Geometry: final body of the model. Coordinates: model frame, mm. Face numbers are marked on the shaded views. A direction names the side the tool comes from. Coordinates: 2 decimals unless noted, no trailing zeros. Loops run counter-clockwise (first coordinate to the right, second up) from the corner with the lowest first, then second, coordinate; pieces in that order, holes last. Notation, with made-up numbers: (34, -23.75) - (74, -23.75) arc R23 ccw to (74, 1.25) - close; hole circle Ø8 at (43.25, 27.25). An arc over 180 degrees is marked (long way). Answer in a Markdown table with one row per item.
from build123d import *

# Parameters (mm, degrees)
F0_W     = 50.8
F0_H     = 50.8
F0_R     = 2.8336716143
F1_DEPTH = 127
F4_R     = 2.3649720561
F5_DEPTH = 50.8
F5_TAPER = 2
F0_W_2   = 43.18
F0_H_2   = 38.1
F6_DEPTH = 41.91


with BuildPart() as f1:
    # F0 (on Top) → F1 (new body)
    with BuildSketch(Plane.XY):
        Rectangle(F0_W, F0_H)
        Circle(F0_R, mode=Mode.SUBTRACT)
    extrude(amount=F1_DEPTH)

    # F2 (on Front) → F3 (revolve)
    with BuildSketch(Plane.XZ):
        with BuildLine():
            Line((0, 108.9572302283), (0, 144.6343966542))
            ThreePointArc((0, 144.6343966542), (-17.8385832129, 126.7958134413), (0, 108.9572302283))
        make_face()
    revolve(axis=Axis((0, 0, 74.6575031662), (0, 0, -1)))

    # F4 (on face) → F5 (join)
    with BuildSketch(Plane.XY.offset(127)):
        Circle(F4_R)
    extrude(amount=F5_DEPTH, taper=F5_TAPER)

    # F0 (on Top) → F6 (join)
    with BuildSketch(Plane.XY):
        Rectangle(F0_W, F0_H)
        Circle(F0_R, mode=Mode.SUBTRACT)
        with Locations((46.99, 0)):
            Rectangle(F0_W_2, F0_H)
        with Locations((46.99, 44.45)):
            Rectangle(F0_W_2, F0_H_2)
    extrude(amount=F6_DEPTH)

    # F7 (on Front) → F8 (revolve)
    with BuildSketch(Plane.XZ):
        with BuildLine():
            Line((44.333525002, 29.0094343104), (44.333525002, 54.918085309))
            ThreePointArc((44.333525002, 54.918085309), (31.3791995027, 41.9637598097), (44.333525002, 29.0094343104))
        make_face()
    revolve(axis=Axis((44.333525002, 0, 30.4748073686), (0, 0, -1)))


solid = f1.part
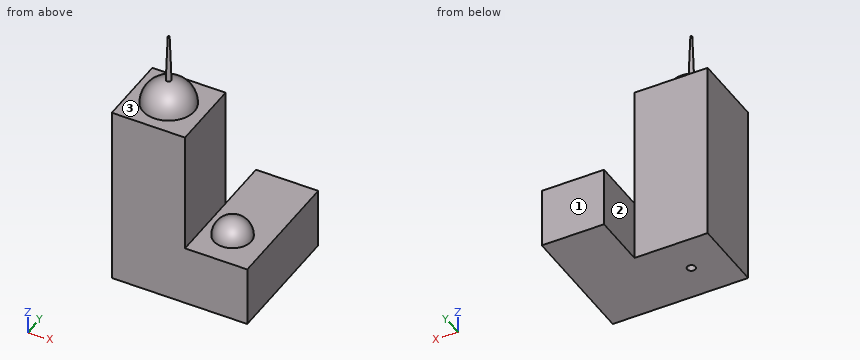
(1) Cut plane A-A on z = 72. Output: boundary loops of the cut face in (x, y), then the cut area to 3 significant figures.
Verdict:
| item | result |
|---|---|
| outline | (-25.4, -25.4) - (25.4, -25.4) - (25.4, 25.4) - (-25.4, 25.4) - close; hole circle Ø5.67 at (0, 0) |
| area | 2,560 mm² |
(2) First-contact query: pin 1 Ø8 at (y, z) = (3.5, 137) entering from +X; pin 2 Ø15 at (x, y) = (12.5, 8.5) entering from +Z; pin 3 Ø2 at (x, z) = (7.5, 27) entering from +Y. Flat tips, straight axial feed; report the tip coordinate or a pass-through.
Verdict:
| item | result |
|---|---|
| pin 1 | stops at x = 16.5 |
| pin 2 | stops at z = 142.93 |
| pin 3 | stops at y = 25.4 |
(3) Cut plane B-B on z = 50. Output: boundary loops of the cut face in (x, y).
Verdict:
| item | result |
|---|---|
| outline | (-25.4, -25.4) - (25.4, -25.4) - (25.4, 25.4) - (-25.4, 25.4) - close; circle Ø20.32 at (44.33, 0); hole circle Ø5.67 at (0, 0) |
(4) Cut plane D-D on y = 35. Output: boundary loops of the cut face in (x, z), then the cut area to 3 significant figures.
Verdict:
| item | result |
|---|---|
| outline | (25.4, 0) - (68.58, 0) - (68.58, 41.91) - (25.4, 41.91) - close |
| area | 1,810 mm² |
(5) Cut plane C-C on x = -8.5. Output: boundary loops of the cut face in (y, z).
Verdict:
| item | result |
|---|---|
| outline | (-25.4, 0) - (25.4, 0) - (25.4, 127) - (15.68, 127) arc R15.68 ccw to (-15.68, 127) - (-25.4, 127) - close |
(6) Ray query, probe 1 along X at (y, z) = (0, 42); probe 2 along Y at (x, z) = (0, 49); probe 3 along X at (y, z) = (0, 49). Return the intervals inside material, ascending.
Verdict:
| item | result |
|---|---|
| probe 1 | x = -25.4 to -2.83, 2.83 to 25.4, 31.38 to 57.29 |
| probe 2 | y = -25.4 to -2.83, 2.83 to 25.4 |
| probe 3 | x = -25.4 to -2.83, 2.83 to 25.4, 33.46 to 55.21 |
(7) Access query for the marked faces 1, 2 and 3. Directions: +Z, -Z, +X, -X, +Y, -Y. A direction counts if a zero-diameter tool reaches every point of the face in a straight line with its end or side. Return the directions, or none.
Verdict:
| item | result |
|---|---|
| face 1 | +Z, -Z, +X, -X, +Y |
| face 2 | +Z, -Z, -X, +Y |
| face 3 | +Z |
